Check sheet for the drawn part. Datum: minimum x, y, z corner. Units: mm. Coordinates: 2 decimals unless noted, no trailing zeros. Write each loop counter-clockwise with the first axis right and the second up, starting at its lowest first coordinate (ties: lowest second). Pieces come first, ordered by that corner, then holes. Notation, with made-up numbers: (-21, 82) -> (3, 82) arc R34 cw to (3, 115) -> close; hole circle Ø7 at (-24, 48.25). An arc over 180 degrees is marked (long way). Write item = value, one per line. Start each with the question number.
(1) Material ranges on probe 1 along X at (y, z) = (76.2, 111.5) (1 decimal); probe 2 along X at (y, z) = (50, 54) (1 decimal); probe 3 along Y at (x, z) = (68.5, 18) (1 decimal), recorded low to high. Write a range as [from, to].
(2) Section check C-C (x = 84.5). Record the cut outline in (y, z), plus the area to 3 significant figures.
(3) Gauge pin test, flat end, axial feed: pin 1 Ø8 at (x, y) = (52.5, 91) entering from +Z. Record the tip position at first contact, or that the pin passes through.
(4) Mould release check, pull along X, two halves, no side actions. Record for the marked faces 1, 2 and 3: released by +X, released by -X, zero draft, split by the parting line, or undercut.
(5) Section check A-A (y = 76.2). Record the cut outline in (x, z) (1 decimal).
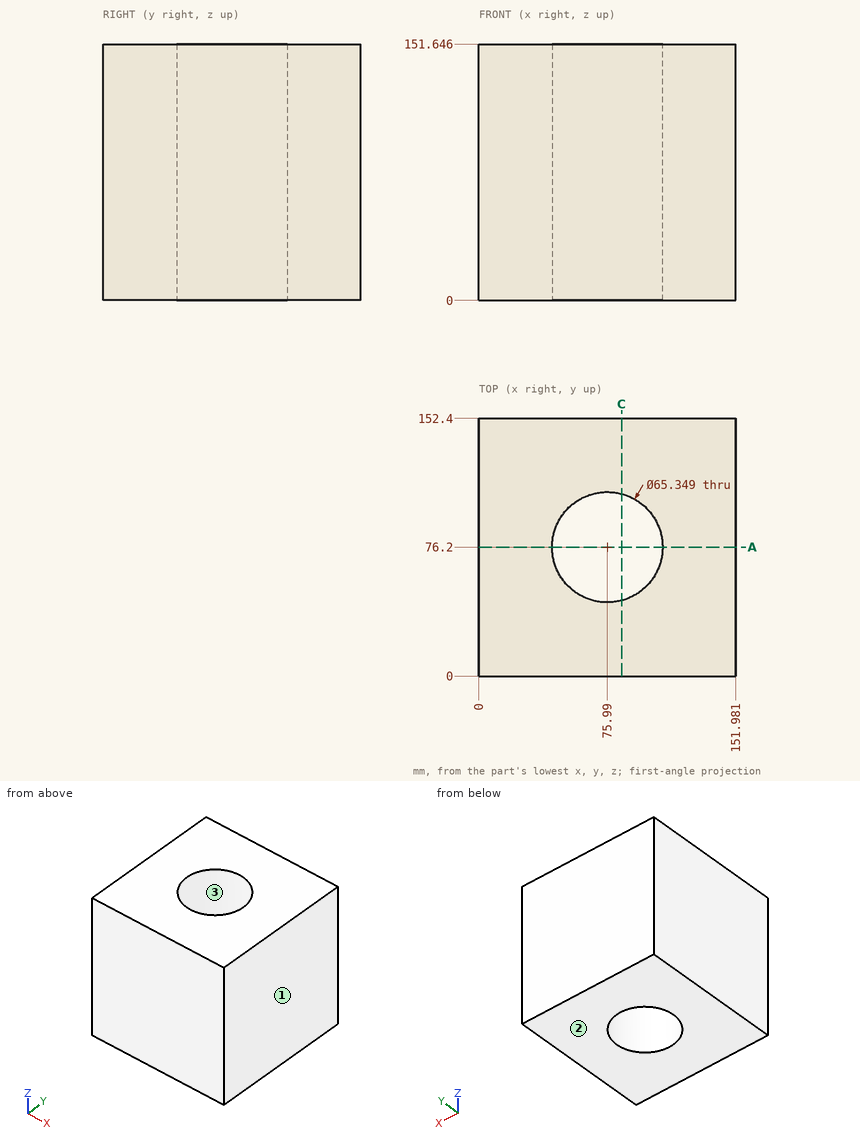
Response:
q1.probe_1 = [0, 43.3], [108.7, 152]
q1.probe_2 = [0, 56.5], [95.5, 152]
q1.probe_3 = [0, 44.4], [108, 152.4]
q2.outline = (0, 0) -> (44.65, 0) -> (44.65, 151.65) -> (0, 151.65) -> close; (107.75, 0) -> (152.4, 0) -> (152.4, 151.65) -> (107.75, 151.65) -> close
q2.area = 13,500 mm2
q3.pin_1 = through
q4.face_1 = released by +X
q4.face_2 = zero draft
q4.face_3 = undercut
q5.outline = (0, 0) -> (43.3, 0) -> (43.3, 151.6) -> (0, 151.6) -> close; (108.7, 0) -> (152, 0) -> (152, 151.6) -> (108.7, 151.6) -> close
